Autodesk Fusion 360 part; units mm, degrees
sketch "Sketch1" plane through (0, 0, 0) normal (0, 0, 1) x (1, 0, 0)
  line L0 (121.4132, 31.9574) -> (124.1913, 31.9574)
  line L1 (124.1913, 31.9574) -> (124.1913, 29.1793)
  line L2 (124.1913, 29.1793) -> (121.4132, 29.1793)
  line L3 (121.4132, 29.1793) -> (121.4132, 31.9574)
  circle A0 centre (122.8023, 30.5684) radius 5.5563
  dimension "d1" = 2.7781
  dimension "d2" = 2.7781
  dimension "d17" = 11.1125
extrude "Extrude1" add sketch "Sketch1" along normal blind 2.3813
extrude "Extrude4" add sketch "Sketch1" along normal blind 2.54 from surface at 2.3813 contours L0 L1 L2 L3 | A0
sketch "Sketch2" plane through (0, 0, 4.9213) normal (0, 0, 1) x (-1, 0, 0)
  line L0 (-124.1913, -29.1793) -> (-121.4132, -29.1793)
  line L1 (-121.4132, -29.1793) -> (-121.4132, -31.9574)
  line L2 (-121.4132, -31.9574) -> (-124.1913, -31.9574)
  line L3 (-124.1913, -31.9574) -> (-124.1913, -29.1793)
  circle A0 centre (-122.8023, -30.5684) radius 3.175
  circle A1 centre (-122.8023, -30.5684) radius 5.5562
  circle A2 centre (-122.8023, -30.5684) radius 5.5562
  point P0 (-121.4132, -30.5684)
  point P1 (-122.8023, -31.9574)
  dimension "d6" = 6.35
extrude "Extrude2" add sketch "Sketch2" along normal blind 6.35 contours L0 L1 L2 L3 | A0
fillet "Fillet1" radius 1.27 1 edges at (125.7624, 31.7165, 11.2712)
sketch "Sketch3" plane through (0, 0, 11.2712) normal (0, 0, 1) x (-1, 0, 0)
  circle A0 centre (-122.8023, -30.5684) radius 1.905
  line L0 (-122.0523, -30.8184) -> (-123.5523, -30.8184) construction
  line L1 (-123.5523, -30.8184) -> (-123.5523, -28.8184)
  line L2 (-123.5523, -28.8184) -> (-122.0523, -28.8184)
  line L3 (-122.0523, -28.8184) -> (-122.0523, -30.8184)
  line L4 (-121.3023, -30.8184) -> (-124.3023, -30.8184)
  line L5 (-124.3023, -30.8184) -> (-122.8023, -32.3184)
  line L6 (-122.8023, -32.3184) -> (-121.3023, -30.8184)
  line L7 (-122.8023, -32.3184) -> (-122.8023, -28.8184) construction
  point P0 (-122.8023, -30.8184)
  point P1 (-122.8023, -30.5684)
  dimension "d11" = 1.5
  dimension "d12" = 2
  dimension "d13" = 1.5
  dimension "d14" = 3
extrude "Extrude3" cut sketch "Sketch3" against normal blind 1 contours L1 L2 L3 L4 | L4 L5 L6
equation "d1 = ( 7 / 64 ) * 1 in"
equation "d2 = ( 7 / 64 ) * 1 in"
equation "d4 = ( 3 / 32 ) * 1 in"
equation "d17 = ( 7 / 16 ) * 1 in"
Here's how the part is built. I have some questions about the finished solid (model axes, mm). A direction names the side the tool comes from. Give positions to 0.01 mm unless a question says otherwise; leave off trailing zeros. Order: outer loops, then holes, each group sorted by start corner. A loop starts at its lowest first (then second) coordinate and runs counter-clockwise, first axis right, second up. Notation, with made-up numbers: M -25,-34 L 25,-34 A15 ccw 25,-25 Z; hole C -17,10 d6. An arc over 180 degrees is marked long. Use a Markdown table: item, result. Add a question column.
1. Suppose I cut it at A-A (z = 10.5). List the corners of the cut face in (x, y) for me, and give its area (3 significant figures).
2. Suppose I cut it at B-B (x = 119.25). List the corners of the cut face in (y, z) for me, and give its area (3 significant figures).
3. For pin 1 Ø3 at (y, z) = (34.5, 8.5) entering from -X; pin 2 Ø1.5 at (x, y) = (118.5, 32.5) entering from +Z; pin 3 Ø1 at (x, z) = (122, 4) entering from -Y, each with a flat end and sliding along its axis, tell me the tip position at first contact or that it passes through.
4. If we mould it in two halves opening along X, with no side actions, what happens to faces 1 (the flat face through (122.063, 31.579, 10.778)), 2 (the cylindrical face through (125.974, 30.708, 7.426)), 3 (the flat face through (125, 31, 0))? For each: +X half, -X half, draft (parallel to the pull), parting line (faces both ways), or undercut.
5. On a 3-axis mill with a long thin cutter (end or side, diameter ignored), from which of +Z, -Z, +X, -X, +Y, -Y can I reach the whole of each face in a straight line? I mean faces 4 (the cylindrical face through (128.102, 28.899, 2.426)), 5 (the flat face through (123, 29.179, 1)), 6 (the flat face through (125, 28, 4.921)). Say none if no direction works.
6. Suppose I cut it at C-C (z = 6.75). List the corners of the cut face in (x, y) for me (3 decimals).
7. Suppose I cut it at D-D (z = 4). List the corners of the cut face in (x, y) for me, and give its area (3 significant figures).
8. I need wall thicknesses on probe 1 along Y at (x, z) = (123, 1.25); probe 2 along Z at (x, y) = (125, 34); probe 3 along Y at (x, z) = (123.5, 1.5). Which ranges of each line are inside material? Lowest first, please. Write a range as from..to.
Results list:
| question | item | result |
|---|---|---|
| 1 | outline | C 122.8,30.57 d6.15; hole M 121.3,30.82 L 122.05,30.82 L 122.05,28.82 L 123.55,28.82 L 123.55,30.82 L 124.3,30.82 L 122.8,32.32 Z |
| 1 | area | 24.4 mm² |
| 2 | outline | M 26.3,0 L 34.84,0 L 34.84,4.92 L 26.3,4.92 Z |
| 2 | area | 42.1 mm² |
| 3 | pin 1 | stops at x = 120.76 |
| 3 | pin 2 | stops at z = 4.92 |
| 3 | pin 3 | stops at y = 25.02 |
| 4 | face 1 | undercut |
| 4 | face 2 | parting line |
| 4 | face 3 | draft |
| 5 | face 4 | +Z, -Z |
| 5 | face 5 | -Z |
| 5 | face 6 | +Z |
| 6 | outline | C 122.802,30.568 d6.35 |
| 7 | outline | C 122.8,30.57 d11.11 |
| 7 | area | 97.0 mm² |
| 8 | probe 1 | y = 25.02..29.18, 31.96..36.12 |
| 8 | probe 2 | z = 0..4.92 |
| 8 | probe 3 | y = 25.06..29.18, 31.96..36.08 |
